Geometry check sheet. Reference: the model listing, model coordinates, mm. Face numbers are marked on the shaded views. A direction names the side the tool comes from. Round coordinates to 2 decimals unless told otherwise and drop trailing zeros. Order: outer loops, then holes, each group sorted by start corner. A loop starts at its lowest first (then second) coordinate and runs counter-clockwise, first axis right, second up. Notation, with made-up numbers: (47.5, -8.75) - (78.5, -8.75) arc R14 ccw to (78.5, 5.25) - close; hole circle Ø4 at (-28, 46). An arc over 180 degrees is marked (long way). Answer as CSV lines item,"result". Start each with the question number.
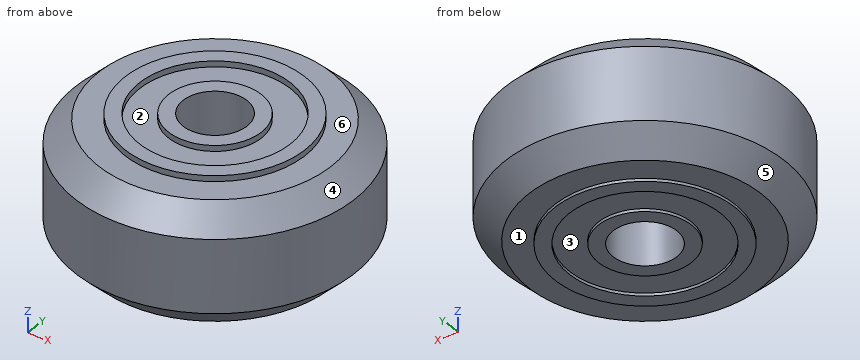
```python
from build123d import *

# Parameters (mm, degrees)
SKETCH1_R                = 12
SKETCH1_R_2              = 7.75
BOSS_EXTRUDE1_DEPTH      = 5.125
CHAMFER1_SIZE            = 2
BOSS_EXTRUDE2_DEPTH      = 0.5
BOSS_EXTRUDE2_DEPTH_BACK = 10.5
SKETCH2_R                = 7.75
SKETCH2_R_2              = 6.5
SKETCH3_R                = 6.5
SKETCH3_R_2              = 4
BOSS_EXTRUDE3_DEPTH      = 10.25
SKETCH4_R                = 4
SKETCH4_R_2              = 2.75
BOSS_EXTRUDE4_DEPTH      = 11


with BuildPart() as part:
    # Sketch1 → Boss-Extrude1 (new, symmetric)
    with BuildSketch(Plane.XY):
        Circle(SKETCH1_R)
        Circle(SKETCH1_R_2, mode=Mode.SUBTRACT)
    extrude(amount=BOSS_EXTRUDE1_DEPTH, both=True)

    # Chamfer1
    chamfer1_edges = [part.edges().sort_by_distance(p)[0] for p in [
        (-12, 0, -5.125),
        (-12, 0, 5.125),
    ]]
    chamfer(chamfer1_edges, length=CHAMFER1_SIZE)

    # Sketch2 → Boss-Extrude2 (add, two sides: drawn at the far end of the back side and taken through both)
    with BuildSketch(Plane.XY.offset(5.125).offset(-BOSS_EXTRUDE2_DEPTH_BACK)):
        Circle(SKETCH2_R)
        Circle(SKETCH2_R_2, mode=Mode.SUBTRACT)
    extrude(amount=BOSS_EXTRUDE2_DEPTH + BOSS_EXTRUDE2_DEPTH_BACK)

    # Sketch3 → Boss-Extrude3 (add)
    with BuildSketch(Plane.XY.offset(5.125)):
        Circle(SKETCH3_R)
        Circle(SKETCH3_R_2, mode=Mode.SUBTRACT)
    extrude(amount=-BOSS_EXTRUDE3_DEPTH)

    # Sketch4 → Boss-Extrude4 (add)
    with BuildSketch(Plane.XY.offset(5.625)):
        Circle(SKETCH4_R)
        Circle(SKETCH4_R_2, mode=Mode.SUBTRACT)
    extrude(amount=-BOSS_EXTRUDE4_DEPTH)


solid = part.part
```
1. Go/stop test with flat-tipped pins: pin 1 Ø4 at (x, y) = (5.5, 9.5) entering from +Z (3 decimals); pin 2 Ø10 at (x, y) = (9, -2.5) entering from -Z (3 decimals); pin 3 Ø6 at (x, z) = (3.5, 4) entering from -Y; pin 4 Ø4 at (x, z) = (5, 0.5) entering from -Y. Record where each tip stops, or that it passes through.
2. Draft check along Y on the marked faces 1, 2, 3 and 4. Enter one of: released by +Y, released by -Y, zero draft, split by the parting line, or undercut.
3. Section check A-A on z = -0.75. Record the boundary of the cut face in (x, y).
4. Access from +Z, -Z, +X, -X, +Y, -Y to the whole of each face (thin tool, end or side, straight path). Record for the marked faces 5 and 6.
5. Thickness scan on probe 1 along Y at (x, z) = (0, 5.4); probe 2 along Y at (x, z) = (0, -0.5); probe 3 along Z at (x, y) = (-4, 8.75) (3 decimals). Record the ranges inside material, lowest first.
Numbers:
1,pin 1,"stops at z = 5.125"
1,pin 2,"stops at z = -5.375"
1,pin 3,"stops at y = -11.98"
1,pin 4,"stops at y = -11.62"
2,face 1,"zero draft"
2,face 2,"undercut"
2,face 3,"undercut"
2,face 4,"split by the parting line"
3,outline,"circle Ø24 at (0, 0); hole circle Ø5.5 at (0, 0)"
4,face 5,"-Z"
4,face 6,"+Z"
5,probe 1,"y = -7.75 to -6.5, -4 to -2.75, 2.75 to 4, 6.5 to 7.75"
5,probe 2,"y = -12 to -2.75, 2.75 to 12"
5,probe 3,"z = -5.125 to 5.125"
